from build123d import *

# Parameters (mm, degrees)
CUT_EXTRUDE1_DEPTH = 21.8
CUT_EXTRUDE2_DEPTH = 39.37


with BuildPart() as part:
    # Sketch2 → Revolve1 (revolve)
    with BuildSketch(Plane.XY):
        Polygon((-10.16, 0), (-4.9911, 0), (-4.9911, -34.29), (-2.032, -34.29), (-2.032, -66.04), (-9.525, -66.04), (-9.525, -25.4), (-12.7, -25.4), (-12.7, -17.78), (-10.16, -17.78), align=None)
    revolve(axis=Axis((0, 0, 0), (0, -1, 0)))

    # Sketch4 → Cut-Extrude1 (cut)
    with BuildSketch(Plane(origin=(0, 0, 0), x_dir=(1, 0, 0), z_dir=(0, 1, 0))):
        with BuildLine():
            Line((1.5, 4.760365449), (1.5, 7.81))
            Line((1.5, 7.81), (-1.5, 7.81))
            Line((-1.5, 7.81), (-1.5, 4.760365449))
            ThreePointArc((-1.5, 4.760365449), (0, 4.9911), (1.5, 4.760365449))
        make_face()
    extrude(amount=-CUT_EXTRUDE1_DEPTH, mode=Mode.SUBTRACT)

    # Sketch5 → Cut-Extrude2 (cut)
    with BuildSketch(Plane.XZ.offset(66.04)):
        with BuildLine():
            Line((-3.175, 8.980256121), (-3.175, 5.805256121))
            Line((-3.175, 5.805256121), (3.175, 5.805256121))
            Line((3.175, 5.805256121), (3.175, 8.980256121))
            ThreePointArc((3.175, 8.980256121), (0, 9.525), (-3.175, 8.980256121))
        make_face()
    extrude(amount=-CUT_EXTRUDE2_DEPTH, mode=Mode.SUBTRACT)


solid = part.part
CAD build for the part. Positions are in the model's coordinates, mm. A direction names the side the tool comes from. Give positions to 0.01 mm unless a question says otherwise; leave off trailing zeros. Write each loop counter-clockwise with the first axis right and the second up, starting at its lowest first coordinate (ties: lowest second). Pieces come first, ordered by that corner, then holes. Notation, with made-up numbers: (88, 52) - (106, 52) arc R20 cw to (106, 91) - close; hole circle Ø3 at (51, 62). An arc over 180 degrees is marked (long way). Answer as CSV lines item,"result".
Q1. Drill centre lines: line 1 (X direction, y = -21.5, z = 0); line 2 (Z direction, x = 0, y = -9). Where is each one in solid material? Low to high. Write a range as from..to.
Result set:
line 1,"-12.7..-4.99, 4.99..12.7"
line 2,"-10.16..-7.81, 4.99..10.16"
Q2. Pull direction X, two halves, no side cores. Call faces 4 (the face through (-0.1, -66.04, -2.5)), 5 (the face through (-1.5, -11, -6)), 6 (the face through (-5.12, -45.44, -8.03)): released by +X, released by -X, zero draft, split by the parting line, or undercut.
Result set:
face 4,"zero draft"
face 5,"undercut"
face 6,"split by the parting line"
Q3. Flat gauge pins, fed straight in: pin 1 Ø1.5 at (y, z) = (-8, -6) entering from -X; pin 2 Ø3 at (x, y) = (1.5, -44) entering from -Z (3 decimals); pin 3 Ø8 at (x, z) = (0, 0) entering from +Y; pin 4 Ø12.5 at (x, z) = (-1.5, 1) entering from +Y. Where does each tip first touch, or does it go through?
Result set:
pin 1,"x = -8.7"
pin 2,"z = -9.525"
pin 3,"y = -34.29"
pin 4,"y = 0"
Q4. Band-saw the part on B-B (x = 0). Give the cut face in (y, z) (3 decimals), and give its area (3 significant figures).
Result set:
outline,"(-66.04, -9.525) - (-25.4, -9.525) - (-25.4, -12.7) - (-17.78, -12.7) - (-17.78, -10.16) - (0, -10.16) - (0, -7.81) - (-21.8, -7.81) - (-21.8, -4.991) - (-34.29, -4.991) - (-34.29, -2.032) - (-66.04, -2.032) - close; (-66.04, 2.032) - (-34.29, 2.032) - (-34.29, 4.991) - (0, 4.991) - (0, 10.16) - (-17.78, 10.16) - (-17.78, 12.7) - (-25.4, 12.7) - (-25.4, 9.525) - (-26.67, 9.525) - (-26.67, 5.805) - (-66.04, 5.805) - close"
area,"650 mm²"
Q5. Band-saw the part on D-D (x = -7.75). Give the cut face in (y, z).
Result set:
outline,"(-66.04, -5.54) - (-25.4, -5.54) - (-25.4, -10.06) - (-17.78, -10.06) - (-17.78, -6.57) - (0, -6.57) - (0, 6.57) - (-17.78, 6.57) - (-17.78, 10.06) - (-25.4, 10.06) - (-25.4, 5.54) - (-66.04, 5.54) - close"
Q6. Band-saw the part on A-A (z = 0). Give the cut face in (x, y) (3 decimals), and give its area (3 significant figures).
Result set:
outline,"(-12.7, -25.4) - (-9.525, -25.4) - (-9.525, -66.04) - (-2.032, -66.04) - (-2.032, -34.29) - (-4.991, -34.29) - (-4.991, 0) - (-10.16, 0) - (-10.16, -17.78) - (-12.7, -17.78) - close; (2.032, -66.04) - (9.525, -66.04) - (9.525, -25.4) - (12.7, -25.4) - (12.7, -17.78) - (10.16, -17.78) - (10.16, 0) - (4.991, 0) - (4.991, -34.29) - (2.032, -34.29) - close"
area,"858 mm²"
Q7. 3-axis set-ups, long thin cutter, end or side, ignore diameter. For faces 1 (the face through (-2, -34.29, 1)), 2 (the face through (5, -25.4, -9)), 3 (the face through (-3.175, -47, 7)): which of +Z, -Z, +X, -X, +Y, -Y reach the whole face in a straight line?
Result set:
face 1,"+Y"
face 2,"-Y"
face 3,"+Z, -Y"
Q8. Band-saw the part on C-C (y = -32). Give the cut face in (x, z) (3 decimals), and give its area (3 significant figures).
Result set:
outline,"(-3.175, 5.805) - (-3.175, 8.98) arc R9.525 ccw (long way) to (3.175, 8.98) - (3.175, 5.805) - close; hole circle Ø9.982 at (0, 0)"
area,"184 mm²"
